Can you work these out from the model? Positions are in its coordinate system, mm. Give positions to 0.01 mm unless a question says otherwise; leave off trailing zeros. Write each loop counter-clockwise with the first axis right and the second up, starting at its lowest first coordinate (ties: lowest second). Pieces come first, ordered by that corner, then holes.
1. If I drill on probe 1 along Z at (x, y) = (0, 3.75); probe 2 along Y at (x, z) = (5, 10.5) (3 decimals), over which ranges is the centre line in solid material (lowest first)?
2. Suppose I cut it at A-A (z = -94). Please give me the cut outline in (x, y) (1 decimal).
3. Suppose I cut it at B-B (x = -21.5). Please give me the cut outline in (y, z) (1 decimal), and give its area (3 significant figures).
4. I'm going to push flat-ended pins straight in: pin 1 (14 mm diameter, centred on y = 8, z = -6, fed in from +X); pin 2 (11.5 mm diameter, centred on y = 8, z = -124, fed in from +X); pin 3 (5 mm diameter, centred on y = 17.5, z = 6, fed in from +X) (3 decimals). Where does each tip first touch, or does it pass through?
5. Suppose I cut it at C-C (z = -35). Please give me the cut outline in (x, y) (1 decimal).
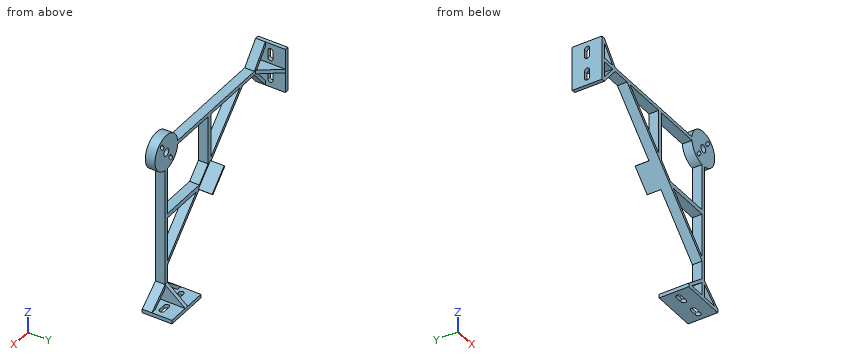
```python
from build123d import *

# Parameters (mm, degrees)
SKETCH1_R                       = 15
BOSS_EXTRUDE2_DEPTH             = 8.255
BOSS_EXTRUDE3_DEPTH             = 8.255
SKETCH5_R                       = 3.249999977
CUT_EXTRUDE3_DEPTH              = 63.5
SKETCH7_W                       = 3.175
SKETCH7_H                       = 25.4
BOSS_EXTRUDE5_DEPTH             = 19.05
CUT_EXTRUDE6_DEPTH              = 149.35
CIRPATTERN2_COUNT               = 2
CIRPATTERN2_ANGLE               = 90
CIRPATTERN3_COUNT               = 2
CIRPATTERN3_ANGLE               = 90
BOSS_EXTRUDE6_DEPTH             = 8.255
BOSS_EXTRUDE7_REACH             = 21.05
BOSS_EXTRUDE7_DIRECTION_2_REACH = 135.35
BOSS_EXTRUDE8_REACH             = 21.05
BOSS_EXTRUDE8_DIRECTION_2_REACH = 135.35
BOSS_EXTRUDE9_REACH             = 133.763
SKETCH19_W                      = 3.81
SKETCH19_H                      = 8.255
BOSS_EXTRUDE10_REACH            = 133.763
SKETCH20_W                      = 3.81
SKETCH20_H                      = 8.255
SKETCH21_W                      = 22.352
SKETCH21_H                      = 20.066
BOSS_EXTRUDE11_DEPTH            = 1.27


with BuildPart() as part:
    # Sketch1 → Boss-Extrude2 (new body)
    with BuildSketch(Plane(origin=(0, 0, 0), x_dir=(1, 0, 0), z_dir=(0, 1, 0))):
        Circle(SKETCH1_R)
    extrude(amount=BOSS_EXTRUDE2_DEPTH)

    # Sketch1<6> → Boss-Extrude3 (add)
    with BuildSketch(Plane(origin=(0, 0, 0), x_dir=(1, 0, 0), z_dir=(0, 1, 0))):
        with BuildLine():
            Line((-1.5875, 130.175), (-1.5875, 14.915758236))
            ThreePointArc((-1.5875, 14.915758236), (0, 15), (1.5875, 14.915758236))
            Line((1.5875, 14.915758236), (1.5875, 130.175))
            Line((1.5875, 130.175), (-1.5875, 130.175))
        make_face()
        with BuildLine():
            ThreePointArc((-14.915758236, -1.5875), (-15, 0), (-14.915758236, 1.5875))
            Line((-14.915758236, 1.5875), (-130.175, 1.5875))
            Line((-130.175, 1.5875), (-130.175, -1.5875))
            Line((-130.175, -1.5875), (-14.915758236, -1.5875))
        make_face()
    extrude(amount=BOSS_EXTRUDE3_DEPTH)

    # Sketch5 → Cut-Extrude3 (cut)
    with BuildSketch(Plane(origin=(0, 8.255, 0), x_dir=(1, 0, 0), z_dir=(0, 1, 0))):
        Circle(SKETCH5_R)
        with BuildLine():
            Line((-5.908712478, 5.423058993), (-7.721732332, 7.873214705))
            ThreePointArc((-7.721732332, 7.873214705), (-7.403164404, 10.004802487), (-5.271576621, 9.686234559))
            Line((-5.271576621, 9.686234559), (-3.458556767, 7.236078848))
            ThreePointArc((-3.458556767, 7.236078848), (-3.777124696, 5.104491065), (-5.908712478, 5.423058993))
        make_face()
        with BuildLine():
            Line((3.458556767, -7.236078848), (5.271576621, -9.686234559))
            ThreePointArc((5.271576621, -9.686234559), (7.403164404, -10.004802487), (7.721732332, -7.873214705))
            Line((7.721732332, -7.873214705), (5.908712478, -5.423058993))
            ThreePointArc((5.908712478, -5.423058993), (3.777124696, -5.104491065), (3.458556767, -7.236078848))
        make_face()
    extrude(amount=-CUT_EXTRUDE3_DEPTH, mode=Mode.SUBTRACT)

    # Sketch7 → Boss-Extrude5 (add, symmetric)
    with BuildSketch(Plane(origin=(0, 0, 0), x_dir=(0, 0, -1), z_dir=(1, 0, 0))):
        with Locations((131.7625, 12.7)):
            Rectangle(SKETCH7_W, SKETCH7_H)
    boss_extrude5 = extrude(amount=BOSS_EXTRUDE5_DEPTH, both=True)

    # Sketch12 → Cut-Extrude6 (cut, through all)
    with BuildSketch(Plane(origin=(0, 0, -133.35), x_dir=(-1, 0, 0), z_dir=(0, 0, -1))):
        with BuildLine():
            Line((-6.35, 10.541), (-12.7, 10.541))
            ThreePointArc((-12.7, 10.541), (-14.859, 12.7), (-12.7, 14.859))
            Line((-12.7, 14.859), (-6.35, 14.859))
            ThreePointArc((-6.35, 14.859), (-4.191, 12.7), (-6.35, 10.541))
        make_face()
        with BuildLine():
            Line((6.35, 14.859), (12.7, 14.859))
            ThreePointArc((12.7, 14.859), (14.859, 12.7), (12.7, 10.541))
            Line((12.7, 10.541), (6.35, 10.541))
            ThreePointArc((6.35, 10.541), (4.191, 12.7), (6.35, 14.859))
        make_face()
    cut_extrude6 = extrude(amount=-CUT_EXTRUDE6_DEPTH, mode=Mode.SUBTRACT)

    # CirPattern2: Boss-Extrude5 ×2 about axis
    cirpattern2_axis = Axis((0, 0, 0), (0, 1, 0))
    for i in range(1, CIRPATTERN2_COUNT):
        add(boss_extrude5.rotate(cirpattern2_axis, i * CIRPATTERN2_ANGLE / (CIRPATTERN2_COUNT - 1)))

    # CirPattern3: Cut-Extrude6 ×2 about axis
    cirpattern3_axis = Axis((0, 0, 0), (0, 1, 0))
    for i in range(1, CIRPATTERN3_COUNT):
        add(cut_extrude6.rotate(cirpattern3_axis, i * CIRPATTERN3_ANGLE / (CIRPATTERN3_COUNT - 1)), mode=Mode.SUBTRACT)

    # Sketch13 → Boss-Extrude6 (add)
    with BuildSketch(Plane.XZ):
        Polygon((-96.628948776, -1.5875), (-1.5875, -96.628948776), (-1.5875, -100.221051224), (-100.221051224, -1.5875), align=None)
        Polygon((-19.05, -130.175), (-1.5875, -115.831500599), (-1.5875, -119.118499401), (-15.048241783, -130.175), align=None)
        Polygon((19.05, -130.175), (1.5875, -115.831500599), (1.5875, -119.118499401), (15.048241783, -130.175), align=None)
        Polygon((-119.118499401, 1.5875), (-130.175, 15.048241783), (-130.175, 19.05), (-115.831500599, 1.5875), align=None)
        Polygon((-119.118499401, -1.5875), (-130.175, -15.048241783), (-130.175, -19.05), (-115.831500599, -1.5875), align=None)
    extrude(amount=-BOSS_EXTRUDE6_DEPTH)

    # Boss-Extrude7: up to this face of the body (flat: up to its plane)
    boss_extrude7_end = Plane(part.part.faces().sort_by_distance((-124.646749701, 4.1275, 1.5875))[0])
    # Sketch14 → Boss-Extrude7 (add, up to the picked face)
    with BuildSketch(Plane.XY, mode=Mode.PRIVATE) as boss_extrude7_sk1:
        Polygon((-130.175, 25.4), (-117.475, 8.255), (-130.175, 8.255), align=None)
    boss_extrude7_tool1 = split(extrude(boss_extrude7_sk1.sketch, amount=BOSS_EXTRUDE7_REACH, mode=Mode.PRIVATE), bisect_by=boss_extrude7_end, keep=Keep.BOTH, mode=Mode.PRIVATE)
    add(boss_extrude7_tool1.solids().sort_by_distance((-125.941667, 13.97, 0))[0])

    # Boss-Extrude7 direction 2: up to this face of the body (flat: up to its plane)
    boss_extrude7_direction_2_end = Plane(part.part.faces().sort_by_distance((-124.646749701, 4.1275, -1.5875))[0])
    # Sketch14 → Boss-Extrude7 direction 2 (add, up to the picked face)
    with BuildSketch(Plane.XY, mode=Mode.PRIVATE) as boss_extrude7_direction_2_sk1:
        Polygon((-130.175, 25.4), (-117.475, 8.255), (-130.175, 8.255), align=None)
    boss_extrude7_direction_2_tool1 = split(extrude(boss_extrude7_direction_2_sk1.sketch, amount=-BOSS_EXTRUDE7_DIRECTION_2_REACH, mode=Mode.PRIVATE), bisect_by=boss_extrude7_direction_2_end, keep=Keep.BOTH, mode=Mode.PRIVATE)
    add(boss_extrude7_direction_2_tool1.solids().sort_by_distance((-125.941667, 13.97, 0))[0])

    # Boss-Extrude8: up to this face of the body (flat: up to its plane)
    boss_extrude8_end = Plane(part.part.faces().sort_by_distance((1.5875, 4.1275, -65.373629417))[0])
    # Sketch15 → Boss-Extrude8 (add, up to the picked face)
    with BuildSketch(Plane(origin=(0, 0, 0), x_dir=(0, 0, -1), z_dir=(1, 0, 0)), mode=Mode.PRIVATE) as boss_extrude8_sk1:
        Polygon((130.175, 25.4), (115.831500599, 8.255), (130.175, 8.255), align=None)
    boss_extrude8_tool1 = split(extrude(boss_extrude8_sk1.sketch, amount=BOSS_EXTRUDE8_REACH, mode=Mode.PRIVATE), bisect_by=boss_extrude8_end, keep=Keep.BOTH, mode=Mode.PRIVATE)
    add(boss_extrude8_tool1.solids().sort_by_distance((0, 13.97, -125.393834))[0])

    # Boss-Extrude8 direction 2: up to this face of the body (flat: up to its plane)
    boss_extrude8_direction_2_end = Plane(part.part.faces().sort_by_distance((-1.5875, 4.1275, -108.026275912))[0])
    # Sketch15 → Boss-Extrude8 direction 2 (add, up to the picked face)
    with BuildSketch(Plane(origin=(0, 0, 0), x_dir=(0, 0, -1), z_dir=(1, 0, 0)), mode=Mode.PRIVATE) as boss_extrude8_direction_2_sk1:
        Polygon((130.175, 25.4), (115.831500599, 8.255), (130.175, 8.255), align=None)
    boss_extrude8_direction_2_tool1 = split(extrude(boss_extrude8_direction_2_sk1.sketch, amount=-BOSS_EXTRUDE8_DIRECTION_2_REACH, mode=Mode.PRIVATE), bisect_by=boss_extrude8_direction_2_end, keep=Keep.BOTH, mode=Mode.PRIVATE)
    add(boss_extrude8_direction_2_tool1.solids().sort_by_distance((0, 13.97, -125.393834))[0])

    # Sketch19 → Boss-Extrude9 (add, up to next)
    with BuildSketch(Plane.ZY.offset(1.5875), mode=Mode.PRIVATE) as boss_extrude9_sk1:
        with Locations((-56.825758236, 4.1275)):
            Rectangle(SKETCH19_W, SKETCH19_H)
    boss_extrude9_tool1 = extrude(boss_extrude9_sk1.sketch, amount=BOSS_EXTRUDE9_REACH, mode=Mode.PRIVATE) - part.part
    add(boss_extrude9_tool1.solids().sort_by_distance((-1.5875, 4.1275, -56.825758))[0])

    # Sketch20 → Boss-Extrude10 (add, up to next)
    with BuildSketch(Plane(origin=(0, 0, -1.5875), x_dir=(-1, 0, 0), z_dir=(0, 0, -1)), mode=Mode.PRIVATE) as boss_extrude10_sk1:
        with Locations((56.825758236, 4.1275)):
            Rectangle(SKETCH20_W, SKETCH20_H)
    boss_extrude10_tool1 = extrude(boss_extrude10_sk1.sketch, amount=BOSS_EXTRUDE10_REACH, mode=Mode.PRIVATE) - part.part
    add(boss_extrude10_tool1.solids().sort_by_distance((-56.825758, 4.1275, -1.5875))[0])

    # Sketch21 → Boss-Extrude11 (add)
    with BuildSketch(Plane(origin=(-50.00625, 0, -50.00625), x_dir=(-0.707106781, 0, 0.707106781), z_dir=(-0.707106781, 0, -0.707106781))):
        with Locations((0, 10.033)):
            Rectangle(SKETCH21_W, SKETCH21_H)
    extrude(amount=BOSS_EXTRUDE11_DEPTH)


solid = part.part
```
Checks:
1. probe 1: z = -133.35 to -3.25, 3.25 to 15
1. probe 2: y = 0 to 8.255
2. outline: (-7.8, 0) - (-4.2, 0) - (-4.2, 8.3) - (-7.8, 8.3) - close; (-1.6, 0) - (1.6, 0) - (1.6, 8.3) - (-1.6, 8.3) - close
3. outline: (0, -80.3) - (8.3, -80.3) - (8.3, -76.7) - (0, -76.7) - close; (0, -58.7) - (8.3, -58.7) - (8.3, -54.9) - (0, -54.9) - close; (0, -1.6) - (8.3, -1.6) - (8.3, 1.6) - (0, 1.6) - close
3. area: 87.3 mm2
4. pin 1: stops at x = 15
4. pin 2: stops at x = 18.53
4. pin 3: stops at x = -130.175
5. outline: (-66.8, 0) - (-63.2, 0) - (-63.2, 8.3) - (-66.8, 8.3) - close; (-58.7, 0) - (-54.9, 0) - (-54.9, 8.3) - (-58.7, 8.3) - close; (-1.6, 0) - (1.6, 0) - (1.6, 8.3) - (-1.6, 8.3) - close
